Check sheet for the modelled part. Datum: model origin and axes. Units: mm. Give positions to 0.01 mm unless a question says otherwise; leave off trailing zeros. Loops run counter-clockwise (first coordinate to the right, second up) from the corner with the lowest first, then second, coordinate; pieces in that order, holes last. Notation, with made-up numbers: (8, 13) - (30, 13) arc R19 ccw to (30, 27) - close; hole circle Ø10 at (32.25, 41.25). An arc over 180 degrees is marked (long way). Answer in a Markdown table with one row per item. Add a question column.
(1) Thickness scan on L1, parallel to Y at x = -0.5, z = 70; L2, parallel to Y at x = 0, z = 78; L3, parallel to X at y = 6, z = 74.5. Record the ranges inside material, lowest first.
(2) Sectioned sample at D-D on y = 15. Enter the section's corners in (x, z), then the cut area to 3 significant figures.
(3) Draft check along Y on faces 1 (the face through (9, -9, 127)), 2 (the face through (-2.71, -12.19, 64.39)), 3 (the face through (-4.52, -20.36, 62.61)). Enter one of: released by +Y, released by -Y, zero draft, split by the parting line, or undercut.
(4) Sectioned sample at C-C on z = 29. Enter the section's corners in (x, y).
(5) Go/stop test with flat-tipped pins: P1, Ø4, axis at y = -5.5, z = 74, coming from the -X side; P2, Ø1.5, axis at y = -14, z = 89, coming from the -X side; P3, Ø12, axis at x = -5.5, z = 32, coming from the +Y side. Record where each tip stops, or that it passes through.
(6) Sectioned sample at A-A on y = 0. Enter the section's corners in (x, z), then the cut area to 3 significant figures.
from build123d import *

# Parameters (mm, degrees)
F0_R     = 20.853702
F1_DEPTH = 127
F2_R     = 9.377492
F3_DEPTH = 127
F4_R     = 12.486205
F5_DEPTH = 127


with BuildPart() as f1:
    # F0 (on Top) → F1 (new body)
    with BuildSketch(Plane.XY):
        Circle(F0_R)
    extrude(amount=F1_DEPTH)

    # F2 (on Top) → F3 (cut)
    with BuildSketch(Plane.XY):
        Circle(F2_R)
    extrude(amount=-F3_DEPTH, mode=Mode.SUBTRACT)

    # F4 (on face) → F5 (cut)
    with BuildSketch(Plane.XY.offset(127)):
        Circle(F4_R)
    extrude(amount=-F5_DEPTH, mode=Mode.SUBTRACT)


solid = f1.part
Reply:
| question | item | result |
|---|---|---|
| 1 | L1 | -20.85 to -12.48, 12.48 to 20.85 |
| 1 | L2 | -20.85 to -12.49, 12.49 to 20.85 |
| 1 | L3 | -19.97 to -10.95, 10.95 to 19.97 |
| 2 | outline | (-14.49, 0) - (14.49, 0) - (14.49, 127) - (-14.49, 127) - close |
| 2 | area | 3,680 mm^2 |
| 3 | face 1 | zero draft |
| 3 | face 2 | undercut |
| 3 | face 3 | split by the parting line |
| 4 | outline | circle Ø41.71 at (0, 0); hole circle Ø24.97 at (0, 0) |
| 5 | P1 | x = -20.56 |
| 5 | P2 | x = -16.1 |
| 5 | P3 | y = 20.85 |
| 6 | outline | (-20.85, 0) - (-12.49, 0) - (-12.49, 127) - (-20.85, 127) - close; (12.49, 0) - (20.85, 0) - (20.85, 127) - (12.49, 127) - close |
| 6 | area | 2,130 mm^2 |
